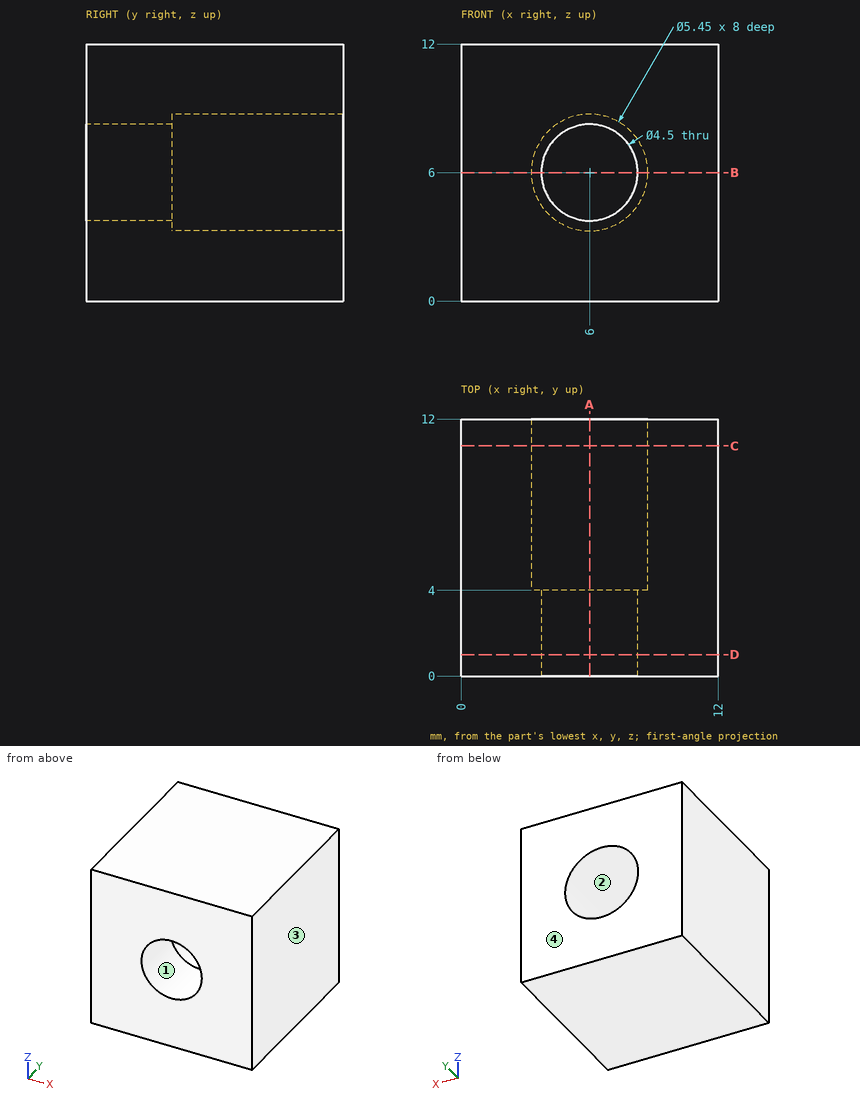
Can you work these out from the drawing? Everything is in mm from the part's minimum corner. Coordinates: 2 decimals unless noted, no trailing zeros. Write each loop counter-clockwise with the first axis right and the second up, starting at its lowest first coordinate (ties: lowest second). Pieces come first, ordered by that corner, then holes. Notation, with made-up numbers: (13, 38.25) -> (52, 38.25) arc R30 ccw to (52, 73.25) -> close; hole circle Ø7 at (-13.5, 77). An arc over 180 degrees is marked (long way). Write item = value, one per line.
(1) For pin 1 (1 mm diameter, centred on y = 5.5, z = 8.5, fed in from -X), with a flat end and sliding along its axis, tell me the tip position at first contact or that it passes through.
Verdict:
pin_1 = 0
(2) Imagine slicing it at D-D (y = 1). Please give me the cut outline in (x, z).
Verdict:
outline = (0, 0) -> (12, 0) -> (12, 12) -> (0, 12) -> close; hole circle Ø4.5 at (6, 6)
(3) Imagine slicing it at B-B (z = 6). Please give me the cut outline in (x, y) (3 decimals).
Verdict:
outline = (0, 0) -> (3.75, 0) -> (3.75, 4) -> (3.275, 4) -> (3.275, 12) -> (0, 12) -> close; (8.25, 0) -> (12, 0) -> (12, 12) -> (8.725, 12) -> (8.725, 4) -> (8.25, 4) -> close
(4) Imagine slicing it at C-C (y = 10.75). Please give me the cut outline in (x, z) (3 decimals), and give its area (3 significant figures).
Verdict:
outline = (0, 0) -> (12, 0) -> (12, 12) -> (0, 12) -> close; hole circle Ø5.45 at (6, 6)
area = 121 mm^2
(5) If I drill on probe 1 along Z at (x, y) = (6, 8.25) (3 decimals); probe 2 along Z at (x, y) = (6, 3.25), over which ranges is the centre line in solid material (lowest first)?
Verdict:
probe_1 = 0 to 3.275, 8.725 to 12
probe_2 = 0 to 3.75, 8.25 to 12
(6) Thinking about a two-plate mould opening in X: for the marked faces 1, 2, 3 and 4, which applies, +X half, -X half, draft (parallel to the pull), parting line (faces both ways), or undercut?
Verdict:
face_1 = undercut
face_2 = undercut
face_3 = +X half
face_4 = draft
(7) Imagine slicing it at A-A (x = 6). Please give me the cut outline in (y, z) (3 decimals), and give its area (3 significant figures).
Verdict:
outline = (0, 0) -> (12, 0) -> (12, 3.275) -> (4, 3.275) -> (4, 3.75) -> (0, 3.75) -> close; (0, 8.25) -> (4, 8.25) -> (4, 8.725) -> (12, 8.725) -> (12, 12) -> (0, 12) -> close
area = 82.4 mm^2
